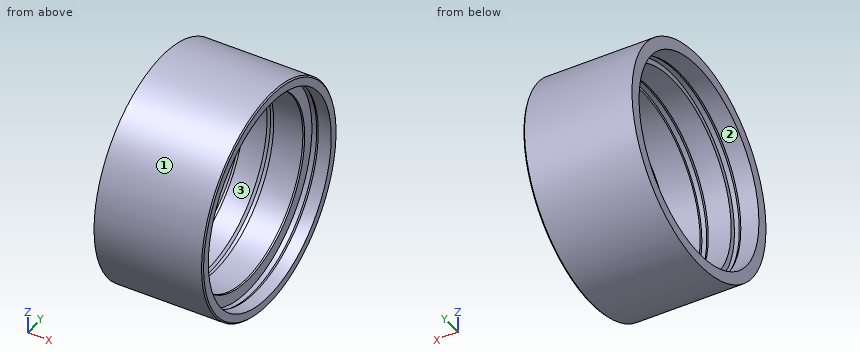
```python
from build123d import *

# Parameters (mm, degrees)
ZKOSEN_1_SIZE = 0.5


with BuildPart() as part:
    # Skica2 → Rotovat1 (revolve)
    with BuildSketch(Plane.XY):
        Polygon((-36.713340937, -44.25), (6, -44.25), (6, -40.6), (0.9, -40.6), (-0.1, -41.25), (-2, -41.25), (-2, -36.5), (-2.716675115, -36.5), (-2.883909622, -37.600000008), (-14.813340937, -37.600000008), (-14.813340937, -38.75), (-16.713340937, -38.75), (-17.713340937, -38.094), (-26.713340937, -38.094), (-26.713340937, -40.25), (-28.613340937, -40.25), (-29.613340937, -39.594), (-36.713340937, -39.594), align=None)
    revolve(axis=Axis((0, 0, 0), (1, 0, 0)))

    # Zkosení1
    zkosen_1_edges = [part.edges().sort_by_distance(p)[0] for p in [
        (6, 44.25, 0),
    ]]
    chamfer(zkosen_1_edges, length=ZKOSEN_1_SIZE)


solid = part.part
```
Geometry check sheet. Reference: the model listing, model coordinates, mm. Face numbers are marked on the shaded views. Coordinates: 2 decimals unless noted, no trailing zeros. Loops run counter-clockwise (first coordinate to the right, second up) from the corner with the lowest first, then second, coordinate; pieces in that order, holes last.
Item 1: Thickness scan on line 1 (Y direction, x = -28, z = 0); line 2 (Z direction, x = -9.75, y = 0); line 3 (Z direction, x = -34.5, y = 0). Record the ranges inside material, lowest first.
Item 2: Release check for a two-part mould opening along Y. For the marked faces 1, 2 and 3 record: released by +Y, released by -Y, zero draft, split by the parting line, or undercut.
Item 3: Go/stop test with flat-tipped pins: pin 1 Ø2 at (x, y) = (-3.5, 6) entering from -Z; pin 2 Ø2 at (x, y) = (-9, -23) entering from -Z; pin 3 Ø5 at (x, z) = (-24.5, -29.5) entering from -Y; pin 4 Ø12 at (y, z) = (-33, -34) entering from +X. Record where each tip stops, or that it passes through.
Item 4: Sectioned sample at B-B, the plane x = -6. Record the boundary of the cut face in (y, z), then the cut area to 3 significant figures.
Item 5: Sectioned sample at A-A, the plane x = -19.5. Record the boundary of the cut face in (y, z).
Check result:
1. line 1: y = -44.25 to -40.25, 40.25 to 44.25
1. line 2: z = -44.25 to -37.6, 37.6 to 44.25
1. line 3: z = -44.25 to -39.59, 39.59 to 44.25
2. face 1: split by the parting line
2. face 2: undercut
2. face 3: undercut
3. pin 1: stops at z = -43.97
3. pin 2: stops at z = -38.39
3. pin 3: stops at y = -35.06
3. pin 4: stops at x = 6
4. outline: circle Ø88.5 at (0, 0); hole circle Ø75.2 at (0, 0)
4. area: 1,710 mm2
5. outline: circle Ø88.5 at (0, 0); hole circle Ø76.19 at (0, 0)
